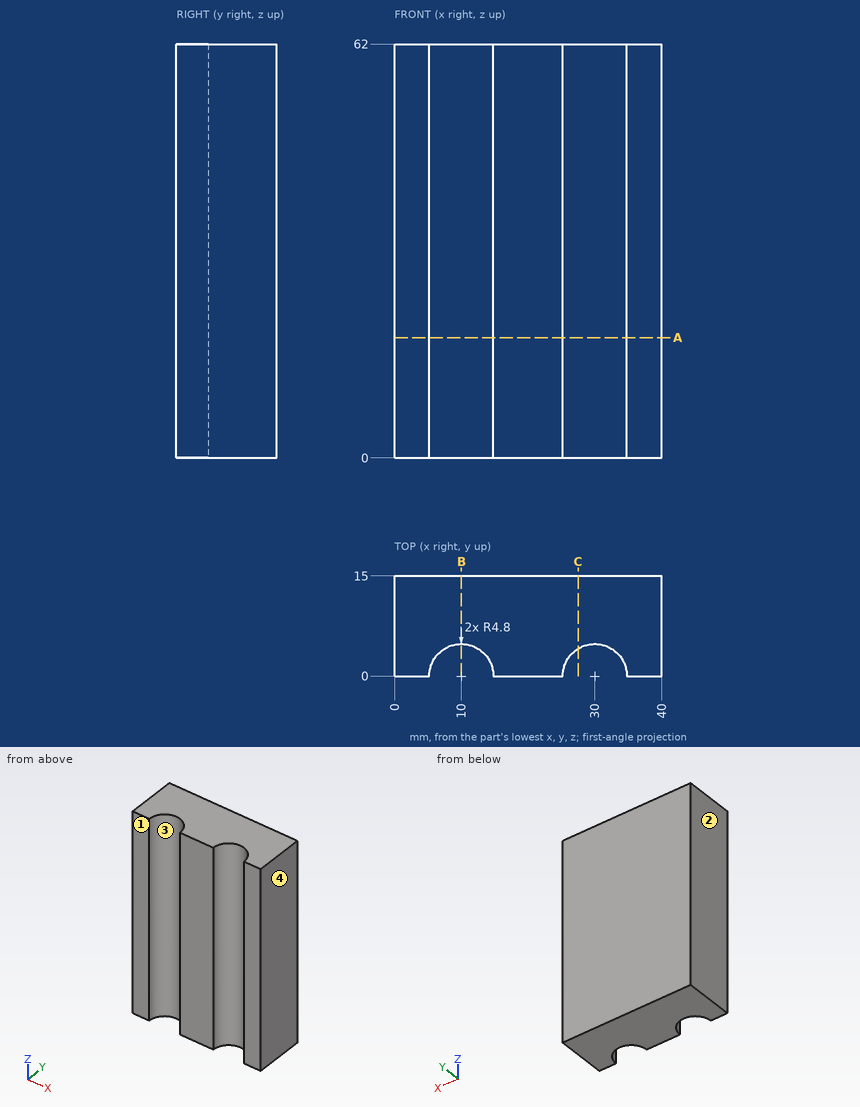
Part print with two shaded views. Sizes in mm from the minimum x, y, z corner. Give positions to 0.01 mm unless a question says otherwise; leave off trailing zeros. Order: outer loops, then holes, each group sorted by start corner. A loop starts at its lowest first (then second) coordinate and runs counter-clockwise, first axis right, second up. Notation, with made-up numbers: M 40.25,25.5 L 69.25,25.5 A25 ccw 69.25,51.5 Z; hole C 13,26.25 d4. An arc over 180 degrees is marked long. Write item = value, one per line.
Q1. Drill centre lines: line 1 (X direction, y = 2, z = 30); line 2 (X direction, y = 3.75, z = 58); line 3 (Y direction, x = 8, z = 15). Where is each one in solid material? Low to high. Write a range as [from, to].
Derived:
line_1 = [0, 5.64], [14.36, 25.64], [34.36, 40]
line_2 = [0, 7], [13, 27], [33, 40]
line_3 = [4.36, 15]
Q2. Cut at A-A, the plane z = 18. List the corners of the cut face in (x, y), then the cut area to 3 significant figures.
Derived:
outline = M 0,0 L 5.2,0 A4.8 cw 14.8,0 L 25.2,0 A4.8 cw 34.8,0 L 40,0 L 40,15 L 0,15 Z
area = 528 mm2
Q3. Cut at C-C, the plane x = 27.5. List the corners of the cut face in (y, z), then the cut area to 3 significant figures.
Derived:
outline = M 4.1,0 L 15,0 L 15,62 L 4.1,62 Z
area = 676 mm2
Q4. Cut at B-B, the plane x = 10. List the corners of the cut face in (y, z), then the cut area to 3 significant figures.
Derived:
outline = M 4.8,0 L 15,0 L 15,62 L 4.8,62 Z
area = 632 mm2
Q5. Two-plate mould, pull along X, no slides. Class the marked faces 1, 2, 3 and 4: pulls with the +X half, pulls with the -X half, needs draft (parallel to the pull), parting line crosses it, or undercut.
Derived:
face_1 = needs draft
face_2 = pulls with the -X half
face_3 = undercut
face_4 = pulls with the +X half
Q6. Flat gauge pins, fed straight in: pin 1 (1 mm diameter, centred on x = 10, y = 10.5, fed in from -Z); pin 2 (4 mm diameter, centred on x = 28, z = 10.5, fed in from -Y). Where does each tip first touch, or does it go through?
Derived:
pin_1 = 0
pin_2 = 2.65
